```python
from build123d import *

# Parameters (mm, degrees)
SKETCH1_R           = 8
SKETCH1_R_2         = 2.625
BOSS_EXTRUDE1_DEPTH = 8
CHAMFER2_SIZE       = 1
CHAMFER3_SIZE       = 1


with BuildPart() as part:
    # Sketch1 → Boss-Extrude1 (new body)
    with BuildSketch(Plane(origin=(0, 0, 0), x_dir=(0, 0, -1), z_dir=(1, 0, 0))):
        Circle(SKETCH1_R)
        Circle(SKETCH1_R_2, mode=Mode.SUBTRACT)
    extrude(amount=BOSS_EXTRUDE1_DEPTH)

    # Chamfer2
    chamfer2_edges = [part.edges().sort_by_distance(p)[0] for p in [
        (0, 0, 2.625),
        (8, 0, 2.625),
    ]]
    chamfer(chamfer2_edges, length=CHAMFER2_SIZE)

    # Chamfer3
    chamfer3_edges = [part.edges().sort_by_distance(p)[0] for p in [
        (0, 0, 8),
    ]]
    chamfer(chamfer3_edges, length=CHAMFER3_SIZE)


solid = part.part
```
Here's how the part is built. I have some questions about the finished solid (model axes, mm). Coordinates: 2 decimals unless noted, no trailing zeros. Write each loop counter-clockwise with the first axis right and the second up, starting at its lowest first coordinate (ties: lowest second). Pieces come first, ordered by that corner, then holes. Notation, with made-up numbers: (39, 0) -> (50, 0) arc R17 cw to (50, 32) -> close; hole circle Ø5 at (-30.75, 3). An arc over 180 degrees is marked (long way). Use a Markdown table: item, result. Add a question column.
(1) Please list where these lines run through material, in increasing order: line 1 (Y direction, x = 3.2, z = 0) (3 decimals); line 2 (Z direction, x = 4, y = 1.25); line 3 (Z direction, x = 4.75, y = 2).
(2) I'm going to push flat-ended pins straight in: P1, Ø3, axis at x = 5, y = 3.5, coming from the -Z side; P2, Ø1, axis at x = 2.5, z = 2, coming from the -Y side; P3, Ø4, axis at y = 0, z = 0, coming from the -X side. Where does each tip first touch, or does it pass through?
(3) We'd pull the mould along Z, two halves only. Please class faces 1 (the flat face through (0, -3, -3)), 2 (the cylindrical face through (4.45, -7.81, 1.73)), 3 (the cylindrical face through (4, 0.8, -2.5)): +Z half, -Z half, draft (parallel to the pull), parting line (faces both ways), or undercut.
(4) If we section it at C-C, the plane x = 4.75: Write out the boundary of the cut face in (y, z) (3 decimals), and give its area (3 significant figures).
(5) If we section it at A-A, the plane z = 0: Write out the boundary of the cut face in (x, y) (3 decimals).
Outcome:
| question | item | result |
|---|---|---|
| 1 | line 1 | y = -8 to -2.625, 2.625 to 8 |
| 1 | line 2 | z = -7.9 to -2.31, 2.31 to 7.9 |
| 1 | line 3 | z = -7.75 to -1.7, 1.7 to 7.75 |
| 2 | P1 | stops at z = -7.75 |
| 2 | P2 | stops at y = -7.86 |
| 2 | P3 | passes through |
| 3 | face 1 | draft |
| 3 | face 2 | parting line |
| 3 | face 3 | undercut |
| 4 | outline | circle Ø16 at (0, 0); hole circle Ø5.25 at (0, 0) |
| 4 | area | 179 mm^2 |
| 5 | outline | (0, -7) -> (1, -8) -> (8, -8) -> (8, -3.625) -> (7, -2.625) -> (1, -2.625) -> (0, -3.625) -> close; (0, 3.625) -> (1, 2.625) -> (7, 2.625) -> (8, 3.625) -> (8, 8) -> (1, 8) -> (0, 7) -> close |
